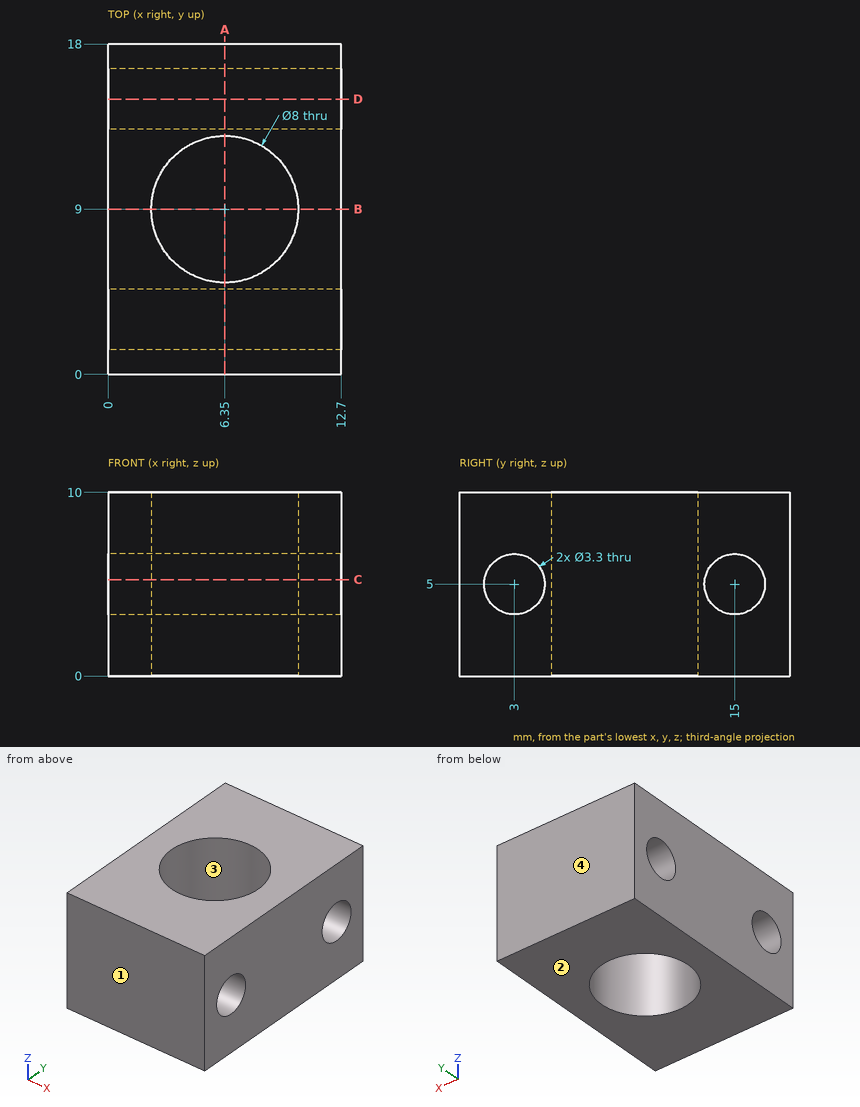
Can you work these out from the drawing? Everything is in mm from the part's minimum corner. Give positions to 0.01 mm unless a question says otherwise; leave off trailing zeros. Loops run counter-clockwise (first coordinate to the right, second up) from the corner with the lowest first, then second, coordinate; pieces in that order, holes last. Notation, with made-up numbers: (34, 82.5) -> (73, 82.5) arc R30 cw to (73, 116.5) -> close; hole circle Ø2 at (55, 56.25). An arc over 180 degrees is marked (long way). Write item = value, one per line.
1) Suppose I cut it at D-D on y = 15. Write out the boundary of the cut face in (x, z), then the cut area to 3 significant figures.
Check result:
outline = (0, 0) -> (12.7, 0) -> (12.7, 3.35) -> (0, 3.35) -> close; (0, 6.65) -> (12.7, 6.65) -> (12.7, 10) -> (0, 10) -> close
area = 85.1 mm2
2) Suppose I cut it at B-B on y = 9. Write out the boundary of the cut face in (x, z).
Check result:
outline = (0, 0) -> (2.35, 0) -> (2.35, 10) -> (0, 10) -> close; (10.35, 0) -> (12.7, 0) -> (12.7, 10) -> (10.35, 10) -> close
3) Suppose I cut it at A-A on x = 6.35. Write out the boundary of the cut face in (y, z), then the cut area to 3 significant figures.
Check result:
outline = (0, 0) -> (5, 0) -> (5, 10) -> (0, 10) -> close; (13, 0) -> (18, 0) -> (18, 10) -> (13, 10) -> close; hole circle Ø3.3 at (3, 5); hole circle Ø3.3 at (15, 5)
area = 82.9 mm2
4) I need wall thicknesses on L1, parallel to Y at x = 11.5, z = 4.25; L2, parallel to Y at x = 5, z = 5; L3, parallel to Y at x = 5.75, z = 5. Which ranges of each line are inside material? Lowest first, please. Write a range as from..to.
Check result:
L1 = 0..1.53, 4.47..13.53, 16.47..18
L2 = 0..1.35, 4.65..5.23, 12.77..13.35, 16.65..18
L3 = 0..1.35, 4.65..5.05, 12.95..13.35, 16.65..18
5) Suppose I cut it at C-C on z = 5.25. Write out the boundary of the cut face in (x, y).
Check result:
outline = (0, 0) -> (12.7, 0) -> (12.7, 1.37) -> (0, 1.37) -> close; (0, 4.63) -> (12.7, 4.63) -> (12.7, 13.37) -> (0, 13.37) -> close; (0, 16.63) -> (12.7, 16.63) -> (12.7, 18) -> (0, 18) -> close; hole circle Ø8 at (6.35, 9)
6) Thinking about a two-plate mould opening in Y: for the marked faces 1, 2, 3 and 4, which applies, released by +Y, released by -Y, zero draft, split by the parting line, or undercut?
Check result:
face_1 = released by -Y
face_2 = zero draft
face_3 = undercut
face_4 = released by +Y
